CAD build for the part. Positions are in the model's coordinates, mm. A direction names the side the tool comes from. Give positions to 0.01 mm unless a question says otherwise; leave off trailing zeros. Write each loop counter-clockwise with the first axis right and the second up, starting at its lowest first coordinate (ties: lowest second). Pieces come first, ordered by that corner, then holes. Notation, with made-up numbers: (26, 68.5) - (39, 68.5) arc R24 ccw to (39, 92.5) - close; hole circle Ø7 at (-20, 9.5). An arc over 180 degrees is marked (long way). Answer as a JSON object with one key per item and string values.
from build123d import *

# Parameters (mm, degrees)
BOSS_EXTRUDE1_DEPTH  = 1.25
SKETCH2_W            = 1
SKETCH2_H            = 0.325
BOSS_EXTRUDE2_DEPTH  = 2
SKETCH3_W            = 1
SKETCH3_H            = 0.325
BOSS_EXTRUDE3_DEPTH  = 2
BOSS_EXTRUDE7_DEPTH  = 1
BOSS_EXTRUDE8_DEPTH  = 1
BOSS_EXTRUDE9_DEPTH  = 7
BOSS_EXTRUDE10_DEPTH = 7


with BuildPart() as part:
    # Sketch1 → Boss-Extrude1 (new body)
    with BuildSketch(Plane.XY):
        Polygon((1, 0), (9, 0), (9, -0.325), (10, -0.325), (10, -1), (17, -1), (17, 1), (10, 1), (0, 1), (-7, 1), (-7, -1), (0, -1), (0, -0.325), (1, -0.325), align=None)
    extrude(amount=BOSS_EXTRUDE1_DEPTH)

    # Sketch2 → Boss-Extrude2 (add)
    with BuildSketch(Plane.XY.offset(1.25)):
        with Locations((0.5, -0.1625)):
            Rectangle(SKETCH2_W, SKETCH2_H)
        with Locations((9.5, -0.1625)):
            Rectangle(SKETCH2_W, SKETCH2_H)
    extrude(amount=BOSS_EXTRUDE2_DEPTH)

    # Sketch3 → Boss-Extrude3 (add)
    with BuildSketch(Plane(origin=(0, 0, 0), x_dir=(-1, 0, 0), z_dir=(0, 0, -1))):
        with Locations((-9.5, -0.1625)):
            Rectangle(SKETCH3_W, SKETCH3_H)
        with Locations((-0.5, -0.1625)):
            Rectangle(SKETCH3_W, SKETCH3_H)
    extrude(amount=BOSS_EXTRUDE3_DEPTH)

    # Sketch7 → Boss-Extrude7 (add)
    with BuildSketch(Plane(origin=(10, 0, 0), x_dir=(0, 0, -1), z_dir=(1, 0, 0))):
        Polygon((-3.25, 0), (-1.25, 1), (-1.25, 0), (-1.25, -0.325), (-3.25, -0.325), align=None)
        Polygon((2, 0), (0, 1), (0, 0), align=None)
    extrude(amount=-BOSS_EXTRUDE7_DEPTH)

    # Sketch8 → Boss-Extrude8 (add)
    with BuildSketch(Plane.ZY):
        Polygon((-2, 0), (0, 1), (0, 0), align=None)
        Polygon((1.25, 1), (1.25, 0), (3.25, 0), align=None)
    extrude(amount=-BOSS_EXTRUDE8_DEPTH)

    # Sketch10 → Boss-Extrude9 (add)
    with BuildSketch(Plane.ZY):
        Polygon((1.25, 1), (3.25, 0), (5.25, -1), (1.25, -1), align=None)
        Polygon((0, 1), (-2, 0), (-4, -1), (0, -1), align=None)
    extrude(amount=BOSS_EXTRUDE9_DEPTH)

    # Sketch11 → Boss-Extrude10 (add)
    with BuildSketch(Plane(origin=(10, 0, 0), x_dir=(0, 0, -1), z_dir=(1, 0, 0))):
        Polygon((-1.25, 1), (-5.25, -1), (-1.25, -1), align=None)
        Polygon((0, 1), (4, -1), (0, -1), align=None)
    extrude(amount=BOSS_EXTRUDE10_DEPTH)


solid = part.part
(1) Saw through at D-D, the plane z = 0.5. Give the cut face in (x, y) (3 decimals).
Answer key:
{"outline": "(-7, -1) - (0, -1) - (0, -0.325) - (1, -0.325) - (1, 0) - (9, 0) - (9, -0.325) - (10, -0.325) - (10, -1) - (17, -1) - (17, 1) - (-7, 1) - close"}
(2) Saw through at B-B, the plane z = -3. Give the cut face in (x, y), and give its area (3 significant figures).
Answer key:
{"outline": "(-7, -1) - (0, -1) - (0, -0.5) - (-7, -0.5) - close; (10, -1) - (17, -1) - (17, -0.5) - (10, -0.5) - close", "area": "7.00 mm²"}
(3) Probe L1, parallel to X at y = -0.8, z = -1.75; L2, parallel to X at y = 0.8, z = 1.5; L3, parallel to Z at x = 7, y = 0.55. List the from-to ranges inside material, lowest first. Write a range as [from, to].
Answer key:
{"L1": "x = [-7, 0], [10, 17]", "L2": "x = [-7, 1], [9, 17]", "L3": "z = [0, 1.25]"}
(4) Flat gauge pins, fed straight in: P1, Ø3, axis at x = -3.5, z = -2, coming from the +Y side; P2, Ø0.8, axis at x = 3, y = 0.5, coming from the -Z side; P3, Ø0.5, axis at x = 4, y = 0.5, coming from the +Z side. Where does each tip first touch, or does it go through?
Answer key:
{"P1": "stops at y = 0.75", "P2": "stops at z = 0", "P3": "stops at z = 1.25"}
(5) Saw through at C-C, the plane x = 9.75. Give the cut face in (y, z) (3 decimals).
Answer key:
{"outline": "(-0.325, -2) - (0, -2) - (1, 0) - (1, 1.25) - (0, 3.25) - (-0.325, 3.25) - close"}
(6) Saw through at A-A, the plane y = -0.65. Give the cut face in (x, z).
Answer key:
{"outline": "(-7, -3.3) - (0, -3.3) - (0, 4.55) - (-7, 4.55) - close; (10, -3.3) - (17, -3.3) - (17, 4.55) - (10, 4.55) - close"}
(7) 3-axis set-ups, long thin cutter, end or side, ignore diameter. For faces 1 (the face through (4.9, 0.5, 1.25)), 2 (the face through (0.5, -0.325, 0.7)), 3 (the face through (4.9, 0.5, 0)), 4 (the face through (13, -1, 1)), 5 (the face through (-3, 0, -2)): which of +Z, -Z, +X, -X, +Y, -Y reach the whole face in a straight line?
Answer key:
{"face 1": "+Z, +Y, -Y", "face 2": "+Z, -Z, -Y", "face 3": "-Z, +Y, -Y", "face 4": "+Z, -Z, +X, -X, -Y", "face 5": "-Z, +X, -X, +Y"}
(8) Pull direction X, two halves, no side cores. Call faces 6 (the face through (0, -0.7, 0.7)), 7 (the face through (13, 0, -2)), 8 (the face through (10, -0.7, 0.7)), 9 (the face through (17, 0, 1)): pulls with the +X half, pulls with the -X half, needs draft (parallel to the pull), parting line crosses it, or undercut.
Answer key:
{"face 6": "undercut", "face 7": "needs draft", "face 8": "undercut", "face 9": "pulls with the +X half"}
